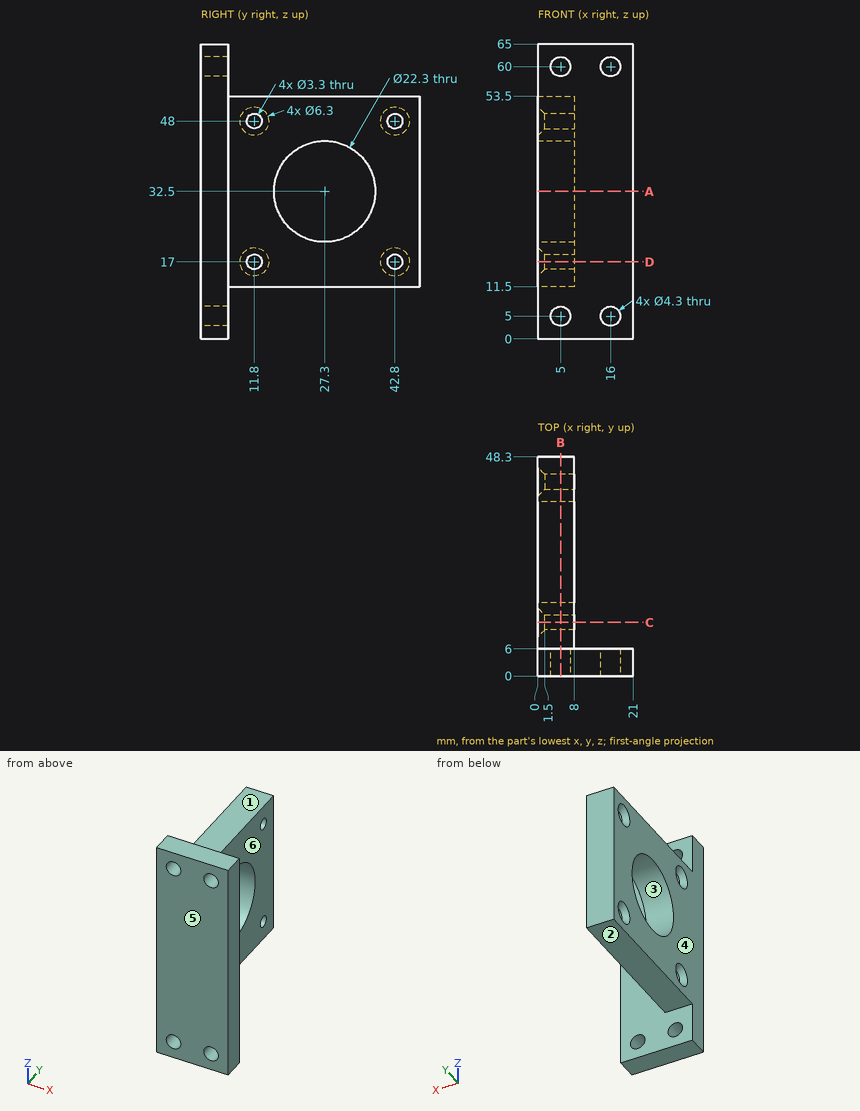
The drawing under review shows one solid part. Ordinate dimensions are in mm from its lowest x, y, z. A direction names the side the tool comes from. Round coordinates to 2 decimals unless told otherwise and drop trailing zeros. Write each loop counter-clockwise with the first axis right and the second up, starting at its lowest first coordinate (ties: lowest second). Pieces come first, ordered by that corner, then holes. Notation, with made-up numbers: M 49,3 L 104,3 A29 cw 104,28 Z; hole C -14,68 d3. An arc over 180 degrees is marked long. One line per item, written item: value. Start each with the question number.
(1) We need section D-D (z = 17). Give the boundary of the cut face in (x, y), and give its area (3 significant figures).
(2) We need section A-A (z = 32.5). Give the boundary of the cut face in (x, y), and give its area (3 significant figures).
(3) Insertion check: pin 1 (6 mm diameter, centred on x = 6, y = 40.5, fed in from +Z); pin 2 (12.5 mm diameter, centred on y = 21, z = 33, fed in from +X); pin 3 (7 mm diameter, centred on x = 5, z = 5, fed in from +Y). Each pin has a flat end and moves straight along its axis. Give the tip position at first contact, or say it passes through.
(4) The part is to be moulded in two halves that separate along Z. For the marked faces 1, 2, 3 and 4, say which applies: released by +Z, released by -Z, zero draft, split by the parting line, or undercut.
(5) Wall thickness on line 1 (Y direction, x = 5.5, z = 17); line 2 (Z direction, x = 5, y = 3.6); line 3 (X direction, y = 5.5, z = 6.5): over which ranges is each line inside the solid? List them lowest first.
(6) We need section C-C (y = 11.8). Give the boundary of the cut face in (x, z), and give its area (3 significant figures).
(7) We need section B-B (x = 5). Give the boundary of the cut face in (y, z), and give its area (3 significant figures).
(8) Machinability: for the marked faces 5 and 6, which of the approach directions +Z, -Z, +X, -X, +Y, -Y give a long, thin tool a straight path to every point of the face, cutting with its end or side? Answer none if there is none.
Result:
1. outline: M 0,0 L 21,0 L 21,6 L 8,6 L 8,10.15 L 1.5,10.15 L 0,8.65 Z; M 0,14.95 L 1.5,13.45 L 8,13.45 L 8,41.15 L 1.5,41.15 L 0,39.65 Z; M 0,45.95 L 1.5,44.45 L 8,44.45 L 8,48.3 L 0,48.3 Z
1. area: 407 mm²
2. outline: M 0,0 L 21,0 L 21,6 L 8,6 L 8,16.15 L 0,16.15 Z; M 0,38.45 L 8,38.45 L 8,48.3 L 0,48.3 Z
2. area: 286 mm²
3. pin 1: z = 53.5
3. pin 2: x = 8
3. pin 3: y = 6
4. face 1: released by +Z
4. face 2: released by -Z
4. face 3: undercut
4. face 4: zero draft
5. line 1: 0 to 10.15, 13.45 to 41.15, 44.45 to 48.3
5. line 2: 0 to 2.85, 7.15 to 57.85, 62.15 to 65
5. line 3: 0 to 3.46, 6.54 to 14.46, 17.54 to 21
6. outline: M 0,11.5 L 8,11.5 L 8,15.35 L 1.5,15.35 L 0,13.85 Z; M 0,20.15 L 1.5,18.65 L 8,18.65 L 8,46.35 L 1.5,46.35 L 0,44.85 Z; M 0,51.15 L 1.5,49.65 L 8,49.65 L 8,53.5 L 0,53.5 Z
6. area: 279 mm²
7. outline: M 0,0 L 6,0 L 6,2.85 L 0,2.85 Z; M 0,7.15 L 6,7.15 L 6,11.5 L 48.3,11.5 L 48.3,53.5 L 6,53.5 L 6,57.85 L 0,57.85 Z; M 0,62.15 L 6,62.15 L 6,65 L 0,65 Z; hole C 11.8,17 d3.3; hole C 11.8,48 d3.3; hole C 27.3,32.5 d22.3; hole C 42.8,17 d3.3; hole C 42.8,48 d3.3
7. area: 1,690 mm²
8. face 5: +Z, -Z, +X, -X, -Y
8. face 6: +Z, -Z, +X, +Y
